```python
from build123d import *

# Parameters (mm, degrees)
SKETCH1_R           = 25.4
BOSS_EXTRUDE1_DEPTH = 25
SKETCH2_R           = 3
CUT_EXTRUDE1_DEPTH  = 44.764369069
SKETCH4_R           = 4
CUT_EXTRUDE4_DEPTH  = 2
SKETCH6_R           = 13
CUT_EXTRUDE6_DEPTH  = 3
SKETCH9_R           = 1.5
CUT_EXTRUDE7_DEPTH  = 5
CUT_EXTRUDE8_START  = -5
SKETCH3_R           = 4
CUT_EXTRUDE8_DEPTH  = 5
CIRPATTERN1_COUNT   = 6


with BuildPart() as part:
    # Sketch1 → Boss-Extrude1 (new body)
    with BuildSketch(Plane.XY):
        Circle(SKETCH1_R)
    extrude(amount=BOSS_EXTRUDE1_DEPTH)

    # Sketch2 → Cut-Extrude1 (cut, through all)
    with BuildSketch(Plane.XY.offset(25)):
        Circle(SKETCH2_R)
    extrude(amount=-CUT_EXTRUDE1_DEPTH, mode=Mode.SUBTRACT)

    # Sketch4 → Cut-Extrude4 (cut)
    with BuildSketch(Plane(origin=(0, 0, 0), x_dir=(-1, 0, 0), z_dir=(0, 0, -1))):
        Circle(SKETCH4_R)
    extrude(amount=-CUT_EXTRUDE4_DEPTH, mode=Mode.SUBTRACT)

    # Sketch6 → Cut-Extrude6 (cut)
    with BuildSketch(Plane.XY.offset(25)):
        Circle(SKETCH6_R)
    extrude(amount=-CUT_EXTRUDE6_DEPTH, mode=Mode.SUBTRACT)

    # Sketch9 → Cut-Extrude7 (cut)
    with BuildSketch(Plane.XY.offset(22)):
        with Locations((0, 8.75)):
            Circle(SKETCH9_R)
    cut_extrude7 = extrude(amount=-CUT_EXTRUDE7_DEPTH, mode=Mode.SUBTRACT)

    # Sketch3 → Cut-Extrude8 (cut)
    with BuildSketch(Plane.XY.offset(25).offset(CUT_EXTRUDE8_START)):
        with Locations(Location((0, 0, 0), (0, 0, 180))):
            Circle(SKETCH3_R)
    extrude(amount=CUT_EXTRUDE8_DEPTH, mode=Mode.SUBTRACT)

    # CirPattern1: Cut-Extrude7 ×6 about axis
    cirpattern1_axis = Axis((0, 0, 0), (0, 0, 1))
    for i in range(1, CIRPATTERN1_COUNT):
        add(cut_extrude7.rotate(cirpattern1_axis, i * 360 / CIRPATTERN1_COUNT), mode=Mode.SUBTRACT)


solid = part.part
```
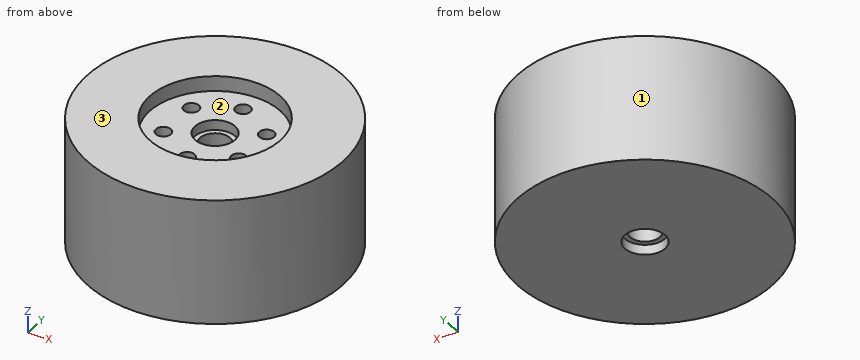
Model file for the job. Use its own axes, mm. Face numbers are marked on the shaded views. Coordinates: 2 decimals unless noted, no trailing zeros. Order: outer loops, then holes, each group sorted by start corner. A loop starts at its lowest first (then second) coordinate and runs counter-clockwise, first axis right, second up. Notation, with made-up numbers: (-4.5, 20) -> (36.5, 20) arc R34 cw to (36.5, 52) -> close; hole circle Ø7 at (-3.75, -13.5). An arc over 180 degrees is marked (long way). Return JSON: item names as keys, results as strings.
Item 1: Mould opens along X. For the marked faces 1, 2 and 3 say: pulls with the +X half, pulls with the -X half, needs draft (parallel to the pull), parting line crosses it, or undercut.
Model answer:
{"face 1": "parting line crosses it", "face 2": "undercut", "face 3": "needs draft"}
Item 2: Slice it at A-A (y = 0). Write the cut outline in (x, z).
Model answer:
{"outline": "(-25.4, 0) -> (-4, 0) -> (-4, 2) -> (-3, 2) -> (-3, 20) -> (-4, 20) -> (-4, 22) -> (-13, 22) -> (-13, 25) -> (-25.4, 25) -> close; (3, 2) -> (4, 2) -> (4, 0) -> (25.4, 0) -> (25.4, 25) -> (13, 25) -> (13, 22) -> (4, 22) -> (4, 20) -> (3, 20) -> close"}
Item 3: Pin check, flat tips, straight feed: P1, Ø3.5, axis at x = 8, y = 4, coming from the +Z side; P2, Ø0.9, axis at x = -7.5, y = -4, coming from the +Z side; P3, Ø2.5, axis at x = 1.5, y = -1.5, coming from the -Z side. Stop position of each tip, or through.
Model answer:
{"P1": "stops at z = 22", "P2": "stops at z = 17", "P3": "stops at z = 2"}
Item 4: Slice it at B-B (x = 0). Write the cut outline in (y, z).
Model answer:
{"outline": "(-25.4, 0) -> (-4, 0) -> (-4, 2) -> (-3, 2) -> (-3, 20) -> (-4, 20) -> (-4, 22) -> (-7.25, 22) -> (-7.25, 17) -> (-10.25, 17) -> (-10.25, 22) -> (-13, 22) -> (-13, 25) -> (-25.4, 25) -> close; (3, 2) -> (4, 2) -> (4, 0) -> (25.4, 0) -> (25.4, 25) -> (13, 25) -> (13, 22) -> (10.25, 22) -> (10.25, 17) -> (7.25, 17) -> (7.25, 22) -> (4, 22) -> (4, 20) -> (3, 20) -> close"}
Item 5: Wall check: line 1 along Y through (x, z) = (0, 21); line 2 along Y through (x, z) = (0, 24.3); line 3 along Y through (x, z) = (0, 6.75). Give the ranges that are in metal, low to high. Write a range as from..to.
Model answer:
{"line 1": "y = -25.4..-10.25, -7.25..-4, 4..7.25, 10.25..25.4", "line 2": "y = -25.4..-13, 13..25.4", "line 3": "y = -25.4..-3, 3..25.4"}
Item 6: Slice it at C-C (z = 7.5). Write the cut outline in (x, y), then the cut area to 3 significant figures.
Model answer:
{"outline": "circle Ø50.8 at (0, 0); hole circle Ø6 at (0, 0)", "area": "2,000 mm²"}
Item 7: Slice it at D-D (y = -8.75). Write the cut outline in (x, z), then the cut area to 3 significant figures.
Model answer:
{"outline": "(-23.85, 0) -> (23.85, 0) -> (23.85, 25) -> (9.61, 25) -> (9.61, 22) -> (1.5, 22) -> (1.5, 17) -> (-1.5, 17) -> (-1.5, 22) -> (-9.61, 22) -> (-9.61, 25) -> (-23.85, 25) -> close", "area": "1,120 mm²"}
